```python
from build123d import *

# Parameters (mm, degrees)
F0_R     = 33.0333203714
F1_DEPTH = 25.4
F2_DEPTH = 7.112
F3_W     = 55.4855957025
F3_H     = 13.38801522
F4_DEPTH = 18.034
F7_DEPTH = 25.4


# Not quite as in the source:
# - a feature names something its author has since deleted; it is built from what else it names


with BuildPart() as f1:
    # F0 (on Top) → F1 (new body)
    with BuildSketch(Plane.XY):
        with BuildLine():
            ThreePointArc((-10.8790392065, -43.5892733327), (27.6552215769, -35.4057476022), (44.9263646842, 0))
            ThreePointArc((44.9263646842, 0), (27.6552215769, 35.4057476022), (-10.8790392065, 43.5892733327))
            ThreePointArc((-10.8790392065, 43.5892733327), (-44.9263646842, 0), (-10.8790392065, -43.5892733327))
        make_face()
        Circle(F0_R, mode=Mode.SUBTRACT)
    extrude(amount=F1_DEPTH)

    # F0 (on Top) → F2 (join)
    with BuildSketch(Plane.XY):
        with BuildLine():
            ThreePointArc((-10.8790392065, -43.5892733327), (27.6552215769, -35.4057476022), (44.9263646842, 0))
            ThreePointArc((44.9263646842, 0), (27.6552215769, 35.4057476022), (-10.8790392065, 43.5892733327))
            ThreePointArc((-10.8790392065, 43.5892733327), (-44.9263646842, 0), (-10.8790392065, -43.5892733327))
        make_face()
        Circle(F0_R, mode=Mode.SUBTRACT)
        with BuildLine():
            ThreePointArc((-10.8790392065, -43.5892733327), (-44.9263646842, 0), (-10.8790392065, 43.5892733327))
            Line((-10.8790392065, 43.5892733327), (-147.3678201437, 43.5892733327))
            Line((-147.3678201437, 43.5892733327), (-147.3678201437, -43.9813993871))
            Line((-147.3678201437, -43.9813993871), (-10.8790392065, -43.5892733327))
        make_face()
    extrude(amount=F2_DEPTH)

    # F3 (on face) → F4 (join)
    with BuildSketch(Plane.XY.offset(7.112)):
        with Locations((-70.6279851798, 6.69400761)):
            Rectangle(F3_W, F3_H)
    extrude(amount=F4_DEPTH)

    # F5 (on face) → F7 (cut)
    with BuildSketch(Plane(origin=(0, 13.38801522, 0), x_dir=(-1, 0, 0), z_dir=(0, 1, 0))):
        Polygon((42.8851873285, 25.146), (98.370783031, 7.112), (98.370783031, 25.146), align=None)
    extrude(amount=-F7_DEPTH, mode=Mode.SUBTRACT)


solid = f1.part
```
Geometry: final body of the model. Coordinates: model frame, mm. A direction names the side the tool comes from. Coordinates: 2 decimals unless noted, no trailing zeros. Write each loop counter-clockwise with the first axis right and the second up, starting at its lowest first coordinate (ties: lowest second). Pieces come first, ordered by that corner, then holes. Notation, with made-up numbers: M 68.5,34.25 L 117.5,34.25 A36 cw 117.5,73.25 Z; hole C 89.5,19.25 d4. An arc over 180 degrees is marked long. Use CSV: the item, a comma, the result in double quotes. Start each with the question number.
1. Cut plane B-B on y = -24.5. Return the cut outline in (x, z).
2. Reachability of faces 4 (the face through (-60, 0, 12)), 5 (the face through (-95, -9, 7.112)), 6 (the face through (-59, 13.388, 12)), 7 (the face through (-78, 43.589, 4)) from +Z, -Z, +X, -X, +Y, -Y: full face, straight path, thin tool, end or side. Return the list, or none.
3. Cut plane D-D on x = -51. Return the cut outline in (y, z).
4. First-contact query: P1, Ø8.5, axis at x = -70.5, z = 14.5, coming from the -Y side; P2, Ø1.5, axis at y = -21.5, z = 10, coming from the -X side; P3, Ø1.5, axis at x = -101.5, y = -5.5, coming from the -Z side; P4, Ø5.5, axis at x = -57, z = 18.5, coming from the +Y side. Flat tips, straight axial feed; report the tip coordinate or a pass-through.
5. Mould query, pull axis X, two halves, no side actions, for faces 1 (the face through (-26.214, -20.1, 12.522)), 2 (the face through (-74, 1, 0)), 3 (the face through (-147.368, 0, 4)). Classes: pulls with the +X half, pulls with the -X half, needs draft (parallel to the pull), parting line crosses it, or undercut.
6. Cut plane A-A on x = 0. Return the cut outline in (y, z).
7. Cut plane C-C on z = 20.25. Return the cut outline in (x, y).
8. Ray query, probe 1 along Y at (x, z) = (0, 14); probe 2 along Z at (x, y) = (-122.5, 21.5); probe 3 along X at (y, z) = (19, 22.5). Return the intervals inside material, ascending.
Entries:
1,outline,"M -147.37,0 L -22.16,0 L -22.16,25.4 L -37.66,25.4 L -37.66,7.11 L -147.37,7.11 Z; M 22.16,0 L 37.66,0 L 37.66,25.4 L 22.16,25.4 Z"
2,face 4,"+Z, -X, -Y"
2,face 5,"+Z, -X"
2,face 6,"+Z, -X, +Y"
2,face 7,"+Z, -Z, -X, +Y"
3,outline,"M -43.7,0 L 43.59,0 L 43.59,7.11 L 13.39,7.11 L 13.39,22.51 L 0,22.51 L 0,7.11 L -43.7,7.11 Z"
4,P1,"y = 0"
4,P2,"x = -39.85"
4,P3,"z = 0"
4,P4,"y = 13.39"
5,face 1,"undercut"
5,face 2,"needs draft"
5,face 3,"pulls with the -X half"
6,outline,"M -44.93,0 L -33.03,0 L -33.03,25.4 L -44.93,25.4 Z; M 33.03,0 L 44.93,0 L 44.93,25.4 L 33.03,25.4 Z"
7,outline,"M -57.95,0 L -44.93,0 A44.93 ccw long -42.89,13.39 L -57.95,13.39 Z; hole C 0,0 d66.07"
8,probe 1,"-44.93 to -33.03, 33.03 to 44.93"
8,probe 2,"0 to 7.11"
8,probe 3,"-40.71 to -27.02, 27.02 to 40.71"
